Print and shaded views of the part. All mm, measured from the part's lowest x, y and z. A direction names the side the tool comes from. Round coordinates to 2 decimals unless told otherwise and drop trailing zeros. Loops run counter-clockwise (first coordinate to the right, second up) from the corner with the lowest first, then second, coordinate; pieces in that order, holes last. Notation, with made-up numbers: (14.25, -16) - (20.25, -16) arc R6 cw to (20.25, -7) - close; hole circle Ø9 at (18.25, -24). An arc over 180 degrees is marked (long way). Answer as a JSON object with one key per item and string values.
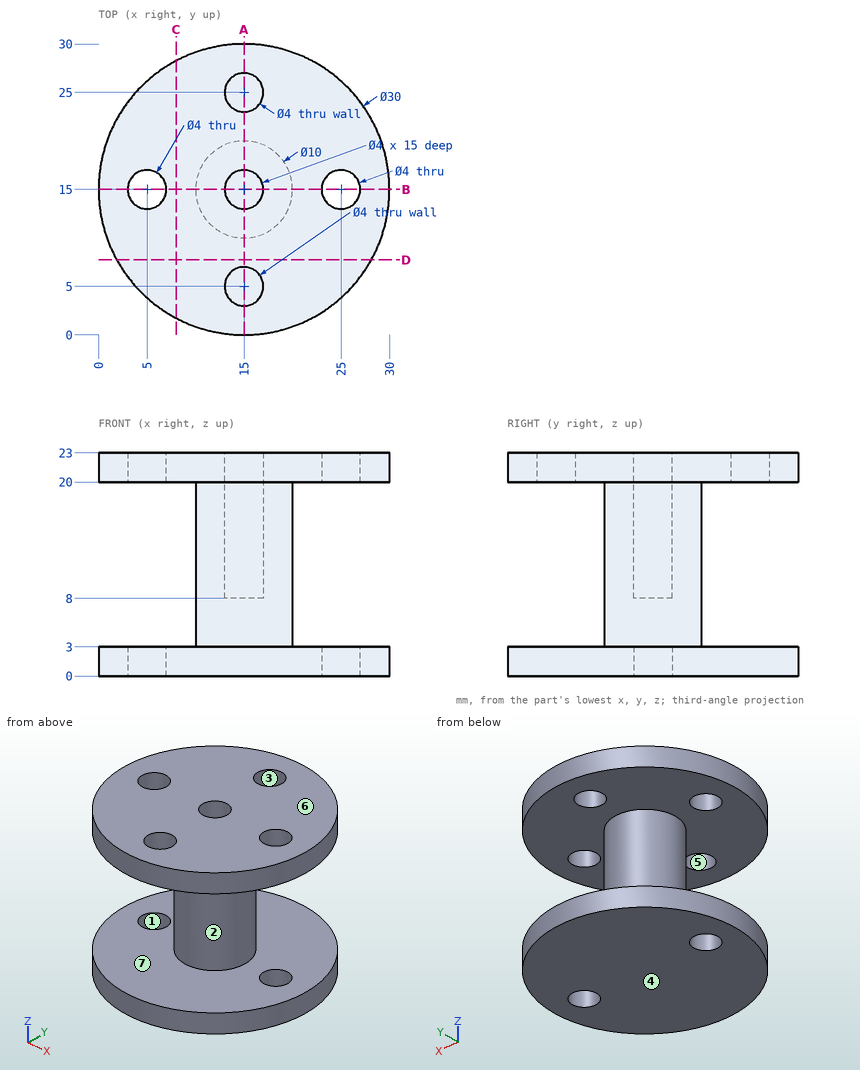
1) Slice it at D-D on y = 7.75. List the corners of the cut face in (x, z), then the cut area to 3 significant figures.
Values follow:
{"outline": "(1.87, 0) - (28.13, 0) - (28.13, 3) - (1.87, 3) - close; (1.87, 20) - (28.13, 20) - (28.13, 23) - (1.87, 23) - close", "area": "158 mm²"}
2) Probe probe 1 along Y at (x, z) = (15, 21.25); probe 2 along Z at (x, y) = (4.75, 11.25); probe 3 along Y at (x, z) = (15, 8.75). List the from-to ranges inside material, lowest first.
Values follow:
{"probe 1": "0 to 3, 7 to 13, 17 to 23, 27 to 30", "probe 2": "0 to 3, 20 to 23", "probe 3": "10 to 13, 17 to 20"}
3) Slice it at C-C on x = 8. List the corners of the cut face in (y, z), then the cut area to 3 significant figures.
Values follow:
{"outline": "(1.73, 0) - (28.27, 0) - (28.27, 3) - (1.73, 3) - close; (1.73, 20) - (28.27, 20) - (28.27, 23) - (1.73, 23) - close", "area": "159 mm²"}
4) Tool access for the marked faces 5, 6 and 7: list every direction of +Z, -Z, +X, -X, +Y, -Y with a clear straight run to the whole face (end or side of a thin tool).
Values follow:
{"face 5": "+Z", "face 6": "+Z, +X, -X, +Y, -Y", "face 7": "none"}
5) Drop flat-ended pins along their axis: P1, Ø3.5, axis at x = 15, y = 25, coming from the +Z side; P2, Ø2, axis at x = 15, y = 15, coming from the +Z side; P3, Ø3.5, axis at x = 25, y = 15, coming from the -Z side; P4, Ø5, axis at x = 9, z = 16, coming from the +Y side. Give the stop position or say it passes through.
Values follow:
{"P1": "z = 3", "P2": "z = 8", "P3": "through", "P4": "y = 18.57"}
6) Slice it at B-B on y = 15. Count the separate pieces of the cut face and the enclosed holes in it, then the cut area to 3 significant figures.
Values follow:
{"separate pieces": "5", "enclosed holes": "0", "area": "242 mm²"}
7) Slice it at A-A on x = 15. List the corners of the cut face in (y, z), then the cut area to 3 significant figures.
Values follow:
{"outline": "(0, 0) - (30, 0) - (30, 3) - (20, 3) - (20, 20) - (23, 20) - (23, 23) - (17, 23) - (17, 8) - (13, 8) - (13, 23) - (7, 23) - (7, 20) - (10, 20) - (10, 3) - (0, 3) - close; (0, 20) - (3, 20) - (3, 23) - (0, 23) - close; (27, 20) - (30, 20) - (30, 23) - (27, 23) - close", "area": "266 mm²"}
8) Two-plate mould, pull along Y, no slides. Class the marked faces 1, 2, 3 and 4: pulls with the +Y half, pulls with the -Y half, needs draft (parallel to the pull), parting line crosses it, or undercut.
Values follow:
{"face 1": "undercut", "face 2": "parting line crosses it", "face 3": "undercut", "face 4": "needs draft"}
